from build123d import *

# Parameters (mm, degrees)
SKETCH_1_R               = 13.5
EXTRUDE_1_DEPTH          = 15
SKETCH_2_R               = 11.75
CUT_EXTRUDE_1_DEPTH      = 11
SKETCH_3_R               = 2
CUT_EXTRUDE_2_DEPTH      = 5
CUT_EXTRUDE_3_DEPTH      = 14.5
CUT_EXTRUDE_3_DEPTH_BACK = 14.5


with BuildPart() as part:
    # Эскиз1 → Бобышка-Вытянуть1 (new body)
    with BuildSketch(Plane(origin=(0, 0, 0), x_dir=(1, 0, 0), z_dir=(0, 1, 0))):
        Circle(SKETCH_1_R)
    extrude(amount=EXTRUDE_1_DEPTH)

    # Эскиз2 → Вырез-Вытянуть1 (cut)
    with BuildSketch(Plane(origin=(0, 15, 0), x_dir=(1, 0, 0), z_dir=(0, 1, 0))):
        Circle(SKETCH_2_R)
    extrude(amount=-CUT_EXTRUDE_1_DEPTH, mode=Mode.SUBTRACT)

    # Эскиз3 → Вырез-Вытянуть2 (cut, through all)
    with BuildSketch(Plane(origin=(0, 4, 0), x_dir=(1, 0, 0), z_dir=(0, 1, 0))):
        with Locations((0, 6.108441075)):
            Circle(SKETCH_3_R)
    extrude(amount=-CUT_EXTRUDE_2_DEPTH, mode=Mode.SUBTRACT)

    # Эскиз4 → Вырез-Вытянуть3 (cut, two sides)
    with BuildSketch(Plane(origin=(0, 0, 0), x_dir=(0, 0, -1), z_dir=(1, 0, 0))) as cut_extrude_3_sk:
        Polygon((2, 5.907484345), (-2, 5.907484345), (-6.083122861, 15), (6.083122861, 15), align=None)
    extrude(amount=CUT_EXTRUDE_3_DEPTH, mode=Mode.SUBTRACT)
    extrude(cut_extrude_3_sk.sketch, amount=-CUT_EXTRUDE_3_DEPTH_BACK, mode=Mode.SUBTRACT)


solid = part.part
Input: part model. Units: mm. Frame: model coordinates. A direction names the side the tool comes from. Round coordinates to 2 decimals unless told otherwise and drop trailing zeros. Order: outer loops, then holes, each group sorted by start corner. A loop starts at its lowest first (then second) coordinate and runs counter-clockwise, first axis right, second up.
1. Set-up query: faces 1 (the face through (5.422, 9.577, 10.424)), 2 (the face through (-0.26, 2.03, -8.09)), 3 (the face through (11.68, 10.52, -4.07)). Return all of +Z, -Z, +X, -X, +Y, -Y with unobstructed straight access to the full face (end or side cutting, diameter ignored); none if empty.
The answers:
face 1: +Y
face 2: +Y, -Y
face 3: +X, -X, +Y
2. Cut plane B-B, the plane x = 0. Output: boundary loops of the cut face in (y, z), then the cut area to 4 significant figures.
The answers:
outline: (0, -13.5) - (15, -13.5) - (15, -11.75) - (4, -11.75) - (4, -8.11) - (0, -8.11) - close; (0, -4.11) - (4, -4.11) - (4, 11.75) - (15, 11.75) - (15, 13.5) - (0, 13.5) - close
area: 130.5 mm2
3. Cut plane D-D, the plane z = -5.25. Output: boundary loops of the cut face in (x, y).
The answers:
outline: (-12.44, 0) - (-1.81, 0) - (-1.81, 4) - (-10.51, 4) - (-10.51, 13.14) - (-12.44, 13.14) - close; (1.81, 0) - (12.44, 0) - (12.44, 13.14) - (10.51, 13.14) - (10.51, 4) - (1.81, 4) - close
4. Mould query, pull axis X, two halves, no side actions, for faces 4 (the face through (0, 4, 0)), 5 (the face through (12.47, 7.4, 5.17)), 6 (the face through (11.679, 10.39, 4.013)). Classes: released by +X, released by -X, zero draft, split by the parting line, or undercut.
The answers:
face 4: undercut
face 5: split by the parting line
face 6: zero draft
5. Cut plane C-C, the plane y = 8.25. Output: boundary loops of the cut face in (x, z), then the cut area to 3 significant figures.
The answers:
outline: (-13.15, -3.05) arc R13.5 ccw to (13.15, -3.05) - (11.35, -3.05) arc R11.75 cw to (-11.35, -3.05) - close; (-13.15, 3.05) - (-11.35, 3.05) arc R11.75 cw to (11.35, 3.05) - (13.15, 3.05) arc R13.5 ccw to start
area: 117 mm2
6. Material intervals for line 1 (Z direction, x = 0, y = 1.85); line 2 (Z direction, x = 0, y = 12.25); line 3 (Y direction, x = -8.75, z = 1.5), sorted ascending.
The answers:
line 1: z = -13.5 to -8.11, -4.11 to 13.5
line 2: z = -13.5 to -11.75, 11.75 to 13.5
line 3: y = 0 to 4
7. Pin query (flat end, axial travel): P1, Ø4, axis at x = 5, y = 7, coming from the -Z side; P2, Ø2, axis at x = 9.5, y = 6.5, coming from the -Z side; P3, Ø2, axis at x = 5, y = 5, coming from the +Z side; P4, Ø6, axis at x = 0, z = 9, coming from the -Y side. Return the tip coordinate at first contact, or that it passes through.
The answers:
P1: stops at z = -13.16
P2: stops at z = -10.49
P3: stops at z = 12.89
P4: stops at y = 0
8. Cut plane A-A, the plane z = 0. Output: boundary loops of the cut face in (x, y), then the cut area to 3 significant figures.
The answers:
outline: (-13.5, 0) - (13.5, 0) - (13.5, 5.91) - (11.75, 5.91) - (11.75, 4) - (-11.75, 4) - (-11.75, 5.91) - (-13.5, 5.91) - close
area: 115 mm2
